from build123d import *

# Parameters (mm, degrees)
SKETCH_1_R      = 1.55
SKETCH_1_R_2    = 1.05
SKETCH_1_W      = 6.5
SKETCH_1_H      = 3.5
SKETCH_1_W_2    = 3.5
SKETCH_1_H_2    = 6.5
SKETCH_1_W_3    = 15.5
SKETCH_1_H_3    = 8.2
EXTRUDE_1_DEPTH = 2.5
FILLET_1_R      = 4
FILLET_2_R      = 7


with BuildPart() as part:
    # 草图1 → 凸台-拉伸1 (new body)
    with BuildSketch(Plane(origin=(0, 0, 0), x_dir=(1, 0, 0), z_dir=(0, 1, 0))):
        with BuildLine():
            Line((114.591143215, 7.468307572), (114.591143215, -7.468307572))
            Line((114.591143215, -7.468307572), (43.193640968, -17.646273029))
            ThreePointArc((43.193640968, -17.646273029), (45.143245402, -33.15226541), (48.27557779, -48.463217404))
            ThreePointArc((48.27557779, -48.463217404), (45.335063646, -55.533708325), (37.709796983, -54.831018053))
            ThreePointArc((37.709796983, -54.831018053), (0, -43.436211003), (-37.709796983, -54.831018053))
            ThreePointArc((-37.709796983, -54.831018053), (-45.335063646, -55.533708325), (-48.27557779, -48.463217404))
            ThreePointArc((-48.27557779, -48.463217404), (-45.143245402, -33.15226541), (-43.193640968, -17.646273029))
            Line((-43.193640968, -17.646273029), (-114.591143215, -7.468307572))
            Line((-114.591143215, -7.468307572), (-114.591143215, 7.468307572))
            Line((-114.591143215, 7.468307572), (-43.193640968, 17.646273029))
            ThreePointArc((-43.193640968, 17.646273029), (-45.143245402, 33.15226541), (-48.27557779, 48.463217404))
            ThreePointArc((-48.27557779, 48.463217404), (-45.335063646, 55.533708325), (-37.709796983, 54.831018053))
            ThreePointArc((-37.709796983, 54.831018053), (0, 43.436211003), (37.709796983, 54.831018053))
            ThreePointArc((37.709796983, 54.831018053), (45.335063646, 55.533708325), (48.27557779, 48.463217404))
            ThreePointArc((48.27557779, 48.463217404), (45.143245402, 33.15226541), (43.193640968, 17.646273029))
            Line((43.193640968, 17.646273029), (114.591143215, 7.468307572))
        make_face()
        with Locations(Location((-36, 43, 0), (0, 0, 270))):
            Circle(SKETCH_1_R, mode=Mode.SUBTRACT)
        with Locations(Location((-32, -42, 0), (0, 0, 270))):
            Circle(SKETCH_1_R, mode=Mode.SUBTRACT)
        with Locations(Location((32, -42, 0), (0, 0, 90))):
            Circle(SKETCH_1_R, mode=Mode.SUBTRACT)
        with Locations(Location((36, 43, 0), (0, 0, 90))):
            Circle(SKETCH_1_R, mode=Mode.SUBTRACT)
        with Locations(Location((42, 50, 0), (0, 0, 270))):
            Circle(SKETCH_1_R, mode=Mode.SUBTRACT)
        with Locations(Location((42, -50, 0), (0, 0, 90))):
            Circle(SKETCH_1_R, mode=Mode.SUBTRACT)
        with Locations(Location((-42, -50, 0), (0, 0, 270))):
            Circle(SKETCH_1_R, mode=Mode.SUBTRACT)
        with Locations(Location((-42, 50, 0), (0, 0, 90))):
            Circle(SKETCH_1_R, mode=Mode.SUBTRACT)
        with Locations(Location((107.7, 0, 0), (0, 0, 270))):
            Circle(SKETCH_1_R_2, mode=Mode.SUBTRACT)
        with Locations(Location((87.3, 0, 0), (0, 0, 270))):
            Circle(SKETCH_1_R_2, mode=Mode.SUBTRACT)
        with Locations(Location((-87.3, 0, 0), (0, 0, 90))):
            Circle(SKETCH_1_R_2, mode=Mode.SUBTRACT)
        with Locations(Location((-107.7, 0, 0), (0, 0, 90))):
            Circle(SKETCH_1_R_2, mode=Mode.SUBTRACT)
        with Locations(Location((70.5, 9, 0), (0, 0, 270))):
            Circle(SKETCH_1_R, mode=Mode.SUBTRACT)
        with Locations(Location((70.5, -9, 0), (0, 0, 90))):
            Circle(SKETCH_1_R, mode=Mode.SUBTRACT)
        with Locations(Location((-70.5, -9, 0), (0, 0, 270))):
            Circle(SKETCH_1_R, mode=Mode.SUBTRACT)
        with Locations(Location((-70.5, 9, 0), (0, 0, 90))):
            Circle(SKETCH_1_R, mode=Mode.SUBTRACT)
        with Locations((-22.25, 39.75)):
            Rectangle(SKETCH_1_W, SKETCH_1_H, mode=Mode.SUBTRACT)
        with Locations((-32.25, 0)):
            Rectangle(SKETCH_1_W_2, SKETCH_1_H_2, mode=Mode.SUBTRACT)
        with Locations((-22.25, -39.75)):
            Rectangle(SKETCH_1_W, SKETCH_1_H, mode=Mode.SUBTRACT)
        with Locations((22.25, 39.75)):
            Rectangle(SKETCH_1_W, SKETCH_1_H, mode=Mode.SUBTRACT)
        with Locations((22.25, -39.75)):
            Rectangle(SKETCH_1_W, SKETCH_1_H, mode=Mode.SUBTRACT)
        with Locations((32.25, 0)):
            Rectangle(SKETCH_1_W_2, SKETCH_1_H_2, mode=Mode.SUBTRACT)
        with BuildLine():
            Line((77.65, -2.176778405), (77.65, -4.025))
            Line((77.65, -4.025), (74.85, -4.025))
            Line((74.85, -4.025), (74.85, -2.176778405))
            ThreePointArc((74.85, -2.176778405), (73.661880176, 0), (74.85, 2.176778405))
            Line((74.85, 2.176778405), (74.85, 4.025))
            Line((74.85, 4.025), (77.65, 4.025))
            Line((77.65, 4.025), (77.65, 2.176778405))
            ThreePointArc((77.65, 2.176778405), (78.838119824, 0), (77.65, -2.176778405))
        make_face(mode=Mode.SUBTRACT)
        with Locations((97.5, 0)):
            Rectangle(SKETCH_1_W_3, SKETCH_1_H_3, mode=Mode.SUBTRACT)
        with Locations((-97.5, 0)):
            Rectangle(SKETCH_1_W_3, SKETCH_1_H_3, mode=Mode.SUBTRACT)
        with BuildLine():
            Line((-74.85, -2.176778405), (-74.85, -4.025))
            Line((-74.85, -4.025), (-77.65, -4.025))
            Line((-77.65, -4.025), (-77.65, -2.176778405))
            ThreePointArc((-77.65, -2.176778405), (-78.838119824, 0), (-77.65, 2.176778405))
            Line((-77.65, 2.176778405), (-77.65, 4.025))
            Line((-77.65, 4.025), (-74.85, 4.025))
            Line((-74.85, 4.025), (-74.85, 2.176778405))
            ThreePointArc((-74.85, 2.176778405), (-73.661880176, 0), (-74.85, -2.176778405))
        make_face(mode=Mode.SUBTRACT)
        with BuildLine():
            Line((-23.978041684, 14.429581723), (-9.54845996, 0))
            Line((-9.54845996, 0), (-23.978041684, -14.429581723))
            ThreePointArc((-23.978041684, -14.429581723), (-26.851664039, -17.042325553), (-29.960234119, -19.370614155))
            ThreePointArc((-29.960234119, -19.370614155), (-27.006361348, 0), (-29.960234119, 19.370614155))
            ThreePointArc((-29.960234119, 19.370614155), (-26.851664039, 17.042325553), (-23.978041684, 14.429581723))
        make_face(mode=Mode.SUBTRACT)
        with BuildLine():
            Line((14.429581723, 23.978041684), (0, 9.54845996))
            Line((0, 9.54845996), (-14.429581723, 23.978041684))
            ThreePointArc((-14.429581723, 23.978041684), (-17.042325553, 26.851664039), (-19.370614155, 29.960234119))
            ThreePointArc((-19.370614155, 29.960234119), (0, 27.006361348), (19.370614155, 29.960234119))
            ThreePointArc((19.370614155, 29.960234119), (17.042325553, 26.851664039), (14.429581723, 23.978041684))
        make_face(mode=Mode.SUBTRACT)
        with BuildLine():
            Line((23.978041684, -14.429581723), (9.54845996, 0))
            Line((9.54845996, 0), (23.978041684, 14.429581723))
            ThreePointArc((23.978041684, 14.429581723), (26.851664039, 17.042325553), (29.960234119, 19.370614155))
            ThreePointArc((29.960234119, 19.370614155), (27.006361348, 0), (29.960234119, -19.370614155))
            ThreePointArc((29.960234119, -19.370614155), (26.851664039, -17.042325553), (23.978041684, -14.429581723))
        make_face(mode=Mode.SUBTRACT)
        with BuildLine():
            Line((-14.429581723, -23.978041684), (0, -9.54845996))
            Line((0, -9.54845996), (14.429581723, -23.978041684))
            ThreePointArc((14.429581723, -23.978041684), (17.042325553, -26.851664039), (19.370614155, -29.960234119))
            ThreePointArc((19.370614155, -29.960234119), (0, -27.006361348), (-19.370614155, -29.960234119))
            ThreePointArc((-19.370614155, -29.960234119), (-17.042325553, -26.851664039), (-14.429581723, -23.978041684))
        make_face(mode=Mode.SUBTRACT)
    extrude(amount=EXTRUDE_1_DEPTH)

    # 圆角1
    fillet_1_edges = [part.edges().sort_by_distance(p)[0] for p in [
        (-114.591143215, 1.25, 7.468307572),
        (-114.591143215, 1.25, -7.468307572),
        (114.591143215, 1.25, -7.468307572),
        (114.591143215, 1.25, 7.468307572),
    ]]
    fillet(fillet_1_edges, radius=FILLET_1_R)

    # 圆角2
    fillet_2_edges = [part.edges().sort_by_distance(p)[0] for p in [
        (-43.193640968, 1.25, 17.646273029),
        (-43.193640968, 1.25, -17.646273029),
        (43.193640968, 1.25, -17.646273029),
        (43.193640968, 1.25, 17.646273029),
    ]]
    fillet(fillet_2_edges, radius=FILLET_2_R)


solid = part.part
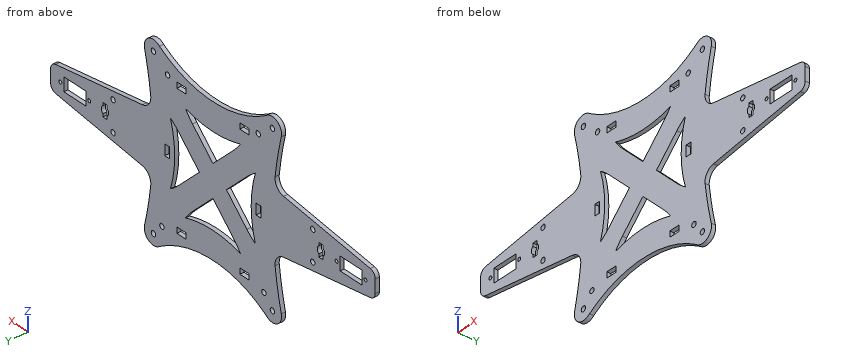
Verification items for the finished model (mm, model axes). Give positions to 0.01 mm unless a question says otherwise; leave off trailing zeros. Write each loop counter-clockwise with the first axis right and the second up, starting at its lowest first coordinate (ties: lowest second). Pieces come first, ordered by that corner, then holes. Notation, with made-up numbers: M 48,-6 L 104,-6 A19 ccw 104,7 Z; hole C 79.25,-2.5 d11. An arc over 180 degrees is marked long. Put each result on its own line as item: value. Start each with the question number.
1. Section check A-A (x = 99.5). Record the cut outline in (y, z).
2. Go/stop test with flat-tipped pins: pin 1 Ø1 at (x, y) = (27, 0.5) entering from +Z; pin 2 Ø0.8 at (y, z) = (2, 39.5) entering from -X; pin 3 Ø1.5 at (x, y) = (-43, 1) entering from +Z. Record where each tip stops, or that it passes through.
3. Section check B-B (y = 0.95). Give the number of separate pieces and of enclosed holes in the cut face, and give its area (3 significant figures).
4. Section check C-C (x = 57.5). Record the cut outline in (y, z), and give its area (3 significant figures).
5. Scan lines: line 1 along Z through (x, y) = (-13, 1.95); line 2 along Z through (x, y) = (-11, 1.75); line 3 along X through (y, z) = (1.35, -43). Record each from-to range of solid material in increasing order. Write a range as [from, to].
Answer list:
1. outline: M 0,-9.62 L 2.5,-9.62 L 2.5,-4.1 L 0,-4.1 Z; M 0,4.1 L 2.5,4.1 L 2.5,9.62 L 0,9.62 Z
2. pin 1: z = 49.24
2. pin 2: x = -46.37
2. pin 3: z = 56.46
3. separate pieces: 1
3. enclosed holes: 30
3. area: 10,400 mm2
4. outline: M 0,-15.61 L 2.5,-15.61 L 2.5,15.61 L 0,15.61 Z
4. area: 78.0 mm2
5. line 1: [-44.69, -28.32], [-22.55, -3.45], [3.45, 22.55], [28.32, 44.69]
5. line 2: [-44.33, -27.94], [-20.55, -1.45], [1.45, 20.55], [27.94, 44.33]
5. line 3: [-47.02, -37.55], [-34.45, 34.45], [37.55, 47.02]
